Work out the finished part from the listing and answer in its coordinate system (mm). A direction names the side the tool comes from. Round coordinates to 2 decimals unless told otherwise and drop trailing zeros. Write each loop counter-clockwise with the first axis right and the second up, starting at its lowest first coordinate (ties: lowest second). Pieces come first, ordered by that corner, then holes. Notation, with made-up numbers: (21, 42) -> (44, 42) arc R27 cw to (44, 81) -> close; hole circle Ø8 at (70, 4.5). An arc over 180 degrees is marked (long way). Answer as a JSON object with one key per item and string values. Group by question number.
from build123d import *

# Parameters (mm, degrees)
F0_W      = 609.6
F0_H      = 863.6
F1_DEPTH  = 1219.2
F2_W      = 609.6
F2_H      = 863.6
F3_DEPTH  = 609.6
F4_W      = 508
F4_H      = 762
F5_DEPTH  = 6.35
F6_W      = 508
F6_H      = 762
F7_DEPTH  = 8.89
F8_W      = 12.7
F8_H      = 127
F9_DEPTH  = 12.7
F10_W     = 12.7
F10_H     = 127
F11_DEPTH = 12.7
F12_W     = 304.8
F12_H     = 304.8
F13_DEPTH = 203.2
F14_W     = 38.1
F14_H     = 38.1
F15_DEPTH = 177.8
F16_W     = 38.1
F16_H     = 38.1
F17_DEPTH = 101.6


with BuildPart() as f1:
    # F0 (on Front) → F1 (new body)
    with BuildSketch(Plane.XZ):
        with Locations((66.055058, 13.796019)):
            Rectangle(F0_W, F0_H)
    extrude(amount=F1_DEPTH)

    # F2 (on face) → F3 (join)
    with BuildSketch(Plane(origin=(-238.744942, 0, 0), x_dir=(0, -1, 0), z_dir=(-1, 0, 0))):
        with Locations((304.8, 13.796019)):
            Rectangle(F2_W, F2_H)
    extrude(amount=F3_DEPTH)

    # F4 (on face) → F5 (join)
    with BuildSketch(Plane(origin=(-238.744942, 0, 0), x_dir=(0, -1, 0), z_dir=(-1, 0, 0))):
        with Locations((914.4, 13.796019)):
            Rectangle(F4_W, F4_H)
    extrude(amount=F5_DEPTH)

    # F6 (on face) → F7 (join)
    with BuildSketch(Plane.XZ.offset(609.6)):
        with Locations((-543.544942, 13.796019)):
            Rectangle(F6_W, F6_H)
    extrude(amount=F7_DEPTH)

    # F8 (on face) → F9 (join)
    with BuildSketch(Plane.XZ.offset(618.49)):
        with Locations((-765.794942, 77.296019)):
            Rectangle(F8_W, F8_H)
    extrude(amount=F9_DEPTH)

    # F10 (on face) → F11 (join)
    with BuildSketch(Plane(origin=(-245.094942, 0, 0), x_dir=(0, -1, 0), z_dir=(-1, 0, 0))):
        with Locations((1136.65, 77.296019)):
            Rectangle(F10_W, F10_H)
    extrude(amount=F11_DEPTH)

    # F12 (on face) → F13 (cut)
    with BuildSketch(Plane.XY.offset(445.596019)):
        with Locations((88.263965, -685.8)):
            Rectangle(F12_W, F12_H)
        with Locations((89.468716, -1016)):
            Rectangle(F12_W, F12_H)
    extrude(amount=-F13_DEPTH, mode=Mode.SUBTRACT)

    # F14 (on face) → F15 (join)
    with BuildSketch(Plane.XY.offset(445.596019)):
        with Locations((269.315895, -844.55)):
            Rectangle(F14_W, F14_H)
    extrude(amount=F15_DEPTH)

    # F16 (on face) → F17 (join)
    with BuildSketch(Plane(origin=(250.265895, 0, 0), x_dir=(0, -1, 0), z_dir=(-1, 0, 0))):
        with Locations((844.55, 604.346019)):
            Rectangle(F16_W, F16_H)
    extrude(amount=F17_DEPTH)


solid = f1.part
1) A cutting plane is placed at A-A on z = 377.5. Determine the outline of the cut face in (x, y).
2) For a pull along X with two mould halves and no side action, classify faces 5 (the face through (-64.136, -688, 345)), 6 (the face through (-95, -466, -418.004)), 7 (the face through (86, -684, 242.396)), 8 (the face through (-848.345, -301, 20)) as released by +X, released by -X, zero draft, split by the parting line, or undercut.
3) A cutting plane is placed at D-D on x = -649. Determine the outline of the cut face in (y, z), plus the area to 3 significant figures.
4) Each of these flat-tipped pins is pushed along its axis until it touches: P1, Ø4, axis at x = -248.5, y = -1139, coming from the -Z side; P2, Ø4, axis at y = -1136, z = 90, coming from the -X side; P3, Ø1, axis at y = -764.5, z = -94.5, coming from the -X side. Where does it stop, or does it pass through?
5) Straight lines are drawn through the part: L1, parallel to Z at x = -289, y = -161.5; L2, parallel to Y at x = -570.5, z = -262.5; L3, parallel to X at y = -629, z = 246.5. For each, find the intervals that lie inside material, in ascending order.
6) A cutting plane is placed at B-B on y = -722.5. Determine the outline of the cut face in (x, z), plus the area to 3 significant figures.
7) A tool of negligible diameter and unlimited length cuts with its end or side. For faces 1 (the face through (87, -1014, 242.396)), 2 (the face through (148.666, -844, 605)), 3 (the face through (251, -825.5, 553)), 4 (the face through (251, -863.6, 553)), from which of +Z, -Z, +X, -X, +Y, -Y can it reach the whole face along a straight path? Write none if from no direction.
8) A cutting plane is placed at C-C on z = 82.5. Determine the outline of the cut face in (x, y), plus the area to 3 significant figures.
Established:
{
 "1": {"outline": "(-848.34, -609.6) -> (-797.54, -609.6) -> (-797.54, -618.49) -> (-289.54, -618.49) -> (-289.54, -609.6) -> (-238.74, -609.6) -> (-238.74, -660.4) -> (-245.09, -660.4) -> (-245.09, -1168.4) -> (-238.74, -1168.4) -> (-238.74, -1219.2) -> (370.86, -1219.2) -> (370.86, 0) -> (-848.34, 0) -> close; hole (-64.14, -838.2) -> (240.66, -838.2) -> (240.66, -533.4) -> (-64.14, -533.4) -> close; hole (-62.93, -1168.4) -> (241.87, -1168.4) -> (241.87, -863.6) -> (-62.93, -863.6) -> close"},
 "2": {"face 5": "undercut", "face 6": "zero draft", "face 7": "undercut", "face 8": "released by -X"},
 "3": {"outline": "(-618.49, -367.2) -> (-609.6, -367.2) -> (-609.6, -418) -> (0, -418) -> (0, 445.6) -> (-609.6, 445.6) -> (-609.6, 394.8) -> (-618.49, 394.8) -> close", "area": "533,000 mm²"},
 "4": {"P1": "stops at z = 13.8", "P2": "stops at x = -257.79", "P3": "stops at x = -245.09"},
 "5": {"L1": "z = -418 to 445.6", "L2": "y = -618.49 to 0", "L3": "x = -238.74 to -64.14, 240.66 to 370.86"},
 "6": {"outline": "(-245.09, -367.2) -> (-238.74, -367.2) -> (-238.74, -418) -> (370.86, -418) -> (370.86, 445.6) -> (240.66, 445.6) -> (240.66, 242.4) -> (-64.14, 242.4) -> (-64.14, 445.6) -> (-238.74, 445.6) -> (-238.74, 394.8) -> (-245.09, 394.8) -> close", "area": "469,000 mm²"},
 "7": {"face 1": "+Z", "face 2": "+Z, -X, +Y, -Y", "face 3": "+Z, +X, -X, +Y", "face 4": "+Z, +X, -X, -Y"},
 "8": {"outline": "(-848.34, -609.6) -> (-797.54, -609.6) -> (-797.54, -618.49) -> (-772.14, -618.49) -> (-772.14, -631.19) -> (-759.44, -631.19) -> (-759.44, -618.49) -> (-289.54, -618.49) -> (-289.54, -609.6) -> (-238.74, -609.6) -> (-238.74, -660.4) -> (-245.09, -660.4) -> (-245.09, -1130.3) -> (-257.79, -1130.3) -> (-257.79, -1143) -> (-245.09, -1143) -> (-245.09, -1168.4) -> (-238.74, -1168.4) -> (-238.74, -1219.2) -> (370.86, -1219.2) -> (370.86, 0) -> (-848.34, 0) -> close", "area": "1,120,000 mm²"}
}
